Check sheet for the modelled part. Datum: model origin and axes. Units: mm. A direction names the side the tool comes from. Give positions to 0.01 mm unless a question says otherwise; leave off trailing zeros. Loops run counter-clockwise (first coordinate to the right, second up) from the corner with the lowest first, then second, coordinate; pieces in that order, holes last. Notation, with made-up numbers: M -37.5,-2 L -5.5,-2 A9 ccw -5.5,4 Z; hole C 40,2 d1. An arc over 180 degrees is marked long. Use one line per item in the form item = value.
Autodesk Inventor part; units mm, degrees
ref_plane "YZ Plane" through (0, 0, 0) normal (1, 0, 0) x (0, 1, 0)
ref_plane "XZ Plane" through (0, 0, 0) normal (0, 1, 0) x (-1, 0, 0)
ref_plane "XY Plane" through (0, 0, 0) normal (0, 0, 1) x (1, 0, 0)
sketch "Szkic1" plane through (0, 0, 0) normal (0, 0, 1) x (1, 0, 0)
  line L0 (9.4719, 9.8006) -> (352.0719, 9.8006)
  line L1 (352.0719, 9.8006) -> (352.0719, -352.7994)
  line L2 (352.0719, -352.7994) -> (9.4719, -352.7994)
  line L3 (9.4719, -352.7994) -> (9.4719, 9.8006)
  point P0 (0, 0)
  point P1 (24.4719, -337.7994)
  point P2 (337.0719, -337.7994)
  point P3 (24.4719, -5.1994)
  point P4 (337.0719, -5.1994)
  dimension "d0" = 342.6
  dimension "d1" = 362.6
  dimension "d4" = 15
  dimension "d5" = 15
  dimension "d6" = 15
  dimension "d7" = 15
  dimension "d8" = 15
  dimension "d9" = 15
  dimension "d10" = 15
  dimension "d11" = 15
  dimension "d19" = 312.6
  dimension "d20" = 332.6
extrude "Wyciągnięcie proste1" add sketch "Szkic1" along normal blind 8
hole "Otwór1" at (24.4719, -337.7994, 0) at (337.0719, -337.7994, 0) at (24.4719, -5.1994, 0) at (337.0719, -5.1994, 0) direction (0, 0, 1) diameter 5 end through all counterbore diameter 10 counterbore depth 4
sketch "Szkic2" plane through (0, 0, 8) normal (0, 0, 1) x (1, 0, 0)
  circle A0 centre (24.4719, -5.1994) radius 2.5
  circle A1 centre (24.4719, -337.7994) radius 2.5
  circle A2 centre (337.0719, -337.7994) radius 2.5
  circle A3 centre (337.0719, -5.1994) radius 2.5
  line L0 (352.0719, 9.8006) -> (9.4719, 9.8006)
  line L1 (9.4719, 9.8006) -> (9.4719, -352.7994)
  line L2 (9.4719, -352.7994) -> (352.0719, -352.7994)
  line L3 (352.0719, -352.7994) -> (352.0719, 9.8006)
  line L4 (39.4719, -20.1994) -> (64.9719, -20.1994)
  line L5 (64.9719, -20.1994) -> (64.9719, -58.3994)
  line L6 (64.9719, -58.3994) -> (39.4719, -58.3994)
  line L7 (39.4719, -58.3994) -> (39.4719, -20.1994)
  line L8 (125.1719, -20.1994) -> (150.6719, -20.1994)
  line L9 (150.6719, -20.1994) -> (150.6719, -58.3994)
  line L10 (150.6719, -58.3994) -> (125.1719, -58.3994)
  line L11 (125.1719, -58.3994) -> (125.1719, -20.1994)
  line L12 (210.8719, -20.1994) -> (236.3719, -20.1994)
  line L13 (236.3719, -20.1994) -> (236.3719, -58.3994)
  line L14 (236.3719, -58.3994) -> (210.8719, -58.3994)
  line L15 (210.8719, -58.3994) -> (210.8719, -20.1994)
  line L16 (296.5719, -20.1994) -> (322.0719, -20.1994)
  line L17 (322.0719, -20.1994) -> (322.0719, -58.3994)
  line L18 (322.0719, -58.3994) -> (296.5719, -58.3994)
  line L19 (296.5719, -58.3994) -> (296.5719, -20.1994)
  line L20 (39.4719, -108.3327) -> (64.9719, -108.3327)
  line L21 (64.9719, -108.3327) -> (64.9719, -146.5327)
  line L22 (64.9719, -146.5327) -> (39.4719, -146.5327)
  line L23 (39.4719, -146.5327) -> (39.4719, -108.3327)
  line L24 (125.1719, -108.3327) -> (150.6719, -108.3327)
  line L25 (150.6719, -108.3327) -> (150.6719, -146.5327)
  line L26 (150.6719, -146.5327) -> (125.1719, -146.5327)
  line L27 (125.1719, -146.5327) -> (125.1719, -108.3327)
  line L28 (210.8719, -108.3327) -> (236.3719, -108.3327)
  line L29 (236.3719, -108.3327) -> (236.3719, -146.5327)
  line L30 (236.3719, -146.5327) -> (210.8719, -146.5327)
  line L31 (210.8719, -146.5327) -> (210.8719, -108.3327)
  line L32 (296.5719, -108.3327) -> (322.0719, -108.3327)
  line L33 (322.0719, -108.3327) -> (322.0719, -146.5327)
  line L34 (322.0719, -146.5327) -> (296.5719, -146.5327)
  line L35 (296.5719, -146.5327) -> (296.5719, -108.3327)
  line L36 (39.4719, -196.4661) -> (64.9719, -196.4661)
  line L37 (64.9719, -196.4661) -> (64.9719, -234.6661)
  line L38 (64.9719, -234.6661) -> (39.4719, -234.6661)
  line L39 (39.4719, -234.6661) -> (39.4719, -196.4661)
  line L40 (125.1719, -196.4661) -> (150.6719, -196.4661)
  line L41 (150.6719, -196.4661) -> (150.6719, -234.6661)
  line L42 (150.6719, -234.6661) -> (125.1719, -234.6661)
  line L43 (125.1719, -234.6661) -> (125.1719, -196.4661)
  line L44 (210.8719, -196.4661) -> (236.3719, -196.4661)
  line L45 (236.3719, -196.4661) -> (236.3719, -234.6661)
  line L46 (236.3719, -234.6661) -> (210.8719, -234.6661)
  line L47 (210.8719, -234.6661) -> (210.8719, -196.4661)
  line L48 (296.5719, -196.4661) -> (322.0719, -196.4661)
  line L49 (322.0719, -196.4661) -> (322.0719, -234.6661)
  line L50 (322.0719, -234.6661) -> (296.5719, -234.6661)
  line L51 (296.5719, -234.6661) -> (296.5719, -196.4661)
  line L52 (39.4719, -284.5994) -> (64.9719, -284.5994)
  line L53 (64.9719, -284.5994) -> (64.9719, -322.7994)
  line L54 (64.9719, -322.7994) -> (39.4719, -322.7994)
  line L55 (39.4719, -322.7994) -> (39.4719, -284.5994)
  line L56 (125.1719, -284.5994) -> (150.6719, -284.5994)
  line L57 (150.6719, -284.5994) -> (150.6719, -322.7994)
  line L58 (150.6719, -322.7994) -> (125.1719, -322.7994)
  line L59 (125.1719, -322.7994) -> (125.1719, -284.5994)
  line L60 (210.8719, -284.5994) -> (236.3719, -284.5994)
  line L61 (236.3719, -284.5994) -> (236.3719, -322.7994)
  line L62 (236.3719, -322.7994) -> (210.8719, -322.7994)
  line L63 (210.8719, -322.7994) -> (210.8719, -284.5994)
  line L64 (296.5719, -284.5994) -> (322.0719, -284.5994)
  line L65 (322.0719, -284.5994) -> (322.0719, -322.7994)
  line L66 (322.0719, -322.7994) -> (296.5719, -322.7994)
  line L67 (296.5719, -322.7994) -> (296.5719, -284.5994)
  point P0 (0, 0)
  dimension "d55" = 362.6
  dimension "d56" = 342.6
  dimension "d57" = 30
  dimension "d58" = 30
  dimension "d61" = 85.7
  dimension "d64" = 88.1333
  dimension "d69" = 25.5
  dimension "d70" = 38.2
extrude "Wyciągnięcie proste2" add sketch "Szkic2" along normal blind 1 contours L4 L5 L6 L7 | L8 L9 L10 L11 | L12 L13 L14 L15 | L16 L17 L18 L19 | L20 L21 L22 L23 | L24 L25 L26 L27 | L28 L29 L30 L31 | L32 L33 L34 L35 | L36 L37 L38 L39 | L40 L41 L42 L43 | L44 L45 L46 L47 | L48 L49 L50 L51 | L52 L53 L54 L55 | L56 L57 L58 L59 | L60 L61 L62 L63 | L64 L65 L66 L67
equation "\"d61\" = -0.666667 * d58 + 0.333333 * d56 - 0.333333 * d69"
equation "\"d64\" = -0.666667 * d57 + 0.333333 * d55 - 0.333333 * d70"
properties part number "CNCM_ALU_8mm_Thick_Heatbed_Plate"
1) Release check for a two-part mould opening along X. For faces 3 (the face through (309, -127, 9)), 4 (the face through (352.072, -169, 4)), 5 (the face through (26, -340, 4)) record: pulls with the +X half, pulls with the -X half, needs draft (parallel to the pull), parting line crosses it, or undercut.
Evaluation:
face_3 = needs draft
face_4 = pulls with the +X half
face_5 = undercut
2) Section check C-C (x = 170.5). Record the cut outline in (y, z), then the cut area to 3 significant figures.
Evaluation:
outline = M -352.8,0 L 9.8,0 L 9.8,8 L -352.8,8 Z
area = 2,900 mm^2
3) Scan lines: line 1 (Y direction, x = 299, z = 8.75); line 2 (Z direction, x = 76, y = -145). Record each from-to range of solid material in increasing order.
Evaluation:
line_1 = -322.8 to -284.6, -234.67 to -196.47, -146.53 to -108.33, -58.4 to -20.2
line_2 = 0 to 8
4) Section check B-B (x = 56.5). Record the cut outline in (y, z), then the cut area to 3 significant figures.
Evaluation:
outline = M -352.8,0 L 9.8,0 L 9.8,8 L -20.2,8 L -20.2,9 L -58.4,9 L -58.4,8 L -108.33,8 L -108.33,9 L -146.53,9 L -146.53,8 L -196.47,8 L -196.47,9 L -234.67,9 L -234.67,8 L -284.6,8 L -284.6,9 L -322.8,9 L -322.8,8 L -352.8,8 Z
area = 3,050 mm^2
5) Set-up check for faces 1 (the face through (52, -303, 9)), 2 (the face through (29.353, -6.283, 2.028)): record each of +Z, -Z, +X, -X, +Y, -Y from which the full face is reachable in a straight line by a thin tool's end or side.
Evaluation:
face_1 = +Z, +X, -X, +Y, -Y
face_2 = -Z
6) Depth check by flat-ended pin: pin 1 Ø6.5 at (x, y) = (337.07, -5.2) entering from -Z; pin 2 Ø2 at (x, y) = (246, -186) entering from +Z; pin 3 Ø0.5 at (x, z) = (138.5, 8.5) entering from +Y. Enter the tip coordinate at first touch or a pass-through.
Evaluation:
pin_1 = 4
pin_2 = 8
pin_3 = -20.2
7) Section check A-A (y = -33.5). Record the cut outline in (x, z).
Evaluation:
outline = M 9.47,0 L 352.07,0 L 352.07,8 L 322.07,8 L 322.07,9 L 296.57,9 L 296.57,8 L 236.37,8 L 236.37,9 L 210.87,9 L 210.87,8 L 150.67,8 L 150.67,9 L 125.17,9 L 125.17,8 L 64.97,8 L 64.97,9 L 39.47,9 L 39.47,8 L 9.47,8 Z
